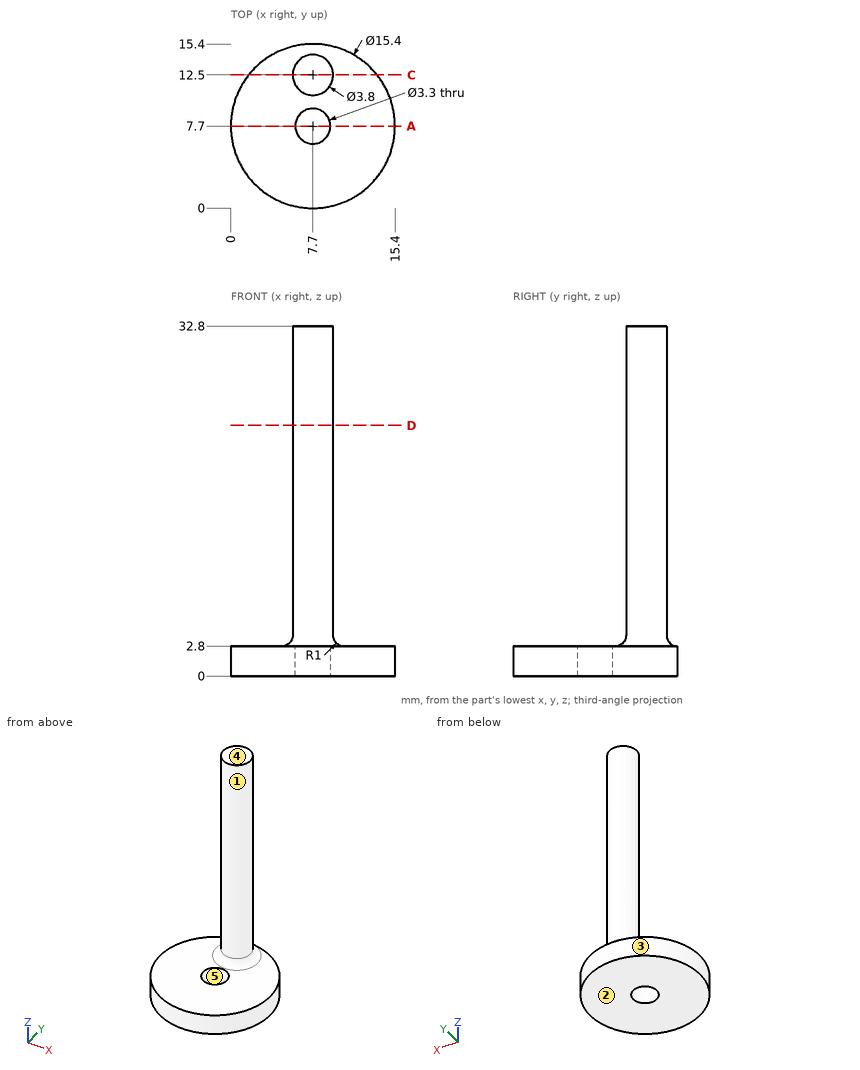
Answer from the drawing. Dimensions are ordinates in mm from the lowest x, y and z of the part. A direction names the side the tool comes from. Give positions to 0.01 mm unless a question says otherwise; leave off trailing zeros. Order: outer loops, then holes, each group sorted by start corner. A loop starts at its lowest first (then second) coordinate and runs counter-clockwise, first axis right, second up. Notation, with made-up numbers: (-18, 67.5) - (35, 67.5) arc R25 ccw to (35, 94.5) - close; hole circle Ø9 at (-30.75, -8.5). An arc over 180 degrees is marked (long way). One line per item, written item: value. Start each with the question number.
1) The mould has two halves that part along X. Classify the marked faces 3, 4 and 5: released by +X, released by -X, zero draft, split by the parting line, or undercut.
2) A tool of negligible diameter and unlimited length cuts with its end or side. For the marked faces 1 and 2, from which of +Z, -Z, +X, -X, +Y, -Y can it reach the whole face along a straight path? Write none if from no direction.
3) Given pin 1 Ø1.5 at (x, z) = (4, 28.5) entering from +Y; pin 2 Ø2 at (x, y) = (2.5, 6) entering from -Z; pin 3 Ø1 at (x, y) = (1.5, 13) entering from +Z, each flat-ended and moving along its own axis, determine where each tip first touches the part or whether it passes through.
4) A cutting plane is placed at C-C on y = 12.5. Give the vertices of the cut face in (x, z).
5) A cutting plane is placed at A-A on y = 7.7. Give the vertices of the cut face in (x, z).
6) Find the intervals of material crossed by L1, parallel to Y at x = 7.7, z = 1.55; L2, parallel to Z at x = 1.5, y = 10; L3, parallel to X at y = 5.75, z = 2, in increasing order.
7) A cutting plane is placed at D-D on z = 23.5. Give the vertices of the cut face in (x, y).
Answer sheet:
1. face 3: split by the parting line
1. face 4: zero draft
1. face 5: undercut
2. face 1: +Z
2. face 2: -Z, +X, -X, +Y, -Y
3. pin 1: passes through
3. pin 2: stops at z = 0
3. pin 3: stops at z = 2.8
4. outline: (1.68, 0) - (13.72, 0) - (13.72, 2.8) - (10.6, 2.8) arc R1 cw to (9.6, 3.8) - (9.6, 32.8) - (5.8, 32.8) - (5.8, 3.8) arc R1 cw to (4.8, 2.8) - (1.68, 2.8) - close
5. outline: (0, 0) - (6.05, 0) - (6.05, 2.8) - (0, 2.8) - close; (9.35, 0) - (15.4, 0) - (15.4, 2.8) - (9.35, 2.8) - close
6. L1: y = 0 to 6.05, 9.35 to 15.4
6. L2: z = 0 to 2.8
6. L3: x = 0.25 to 15.15
7. outline: circle Ø3.8 at (7.7, 12.5)
